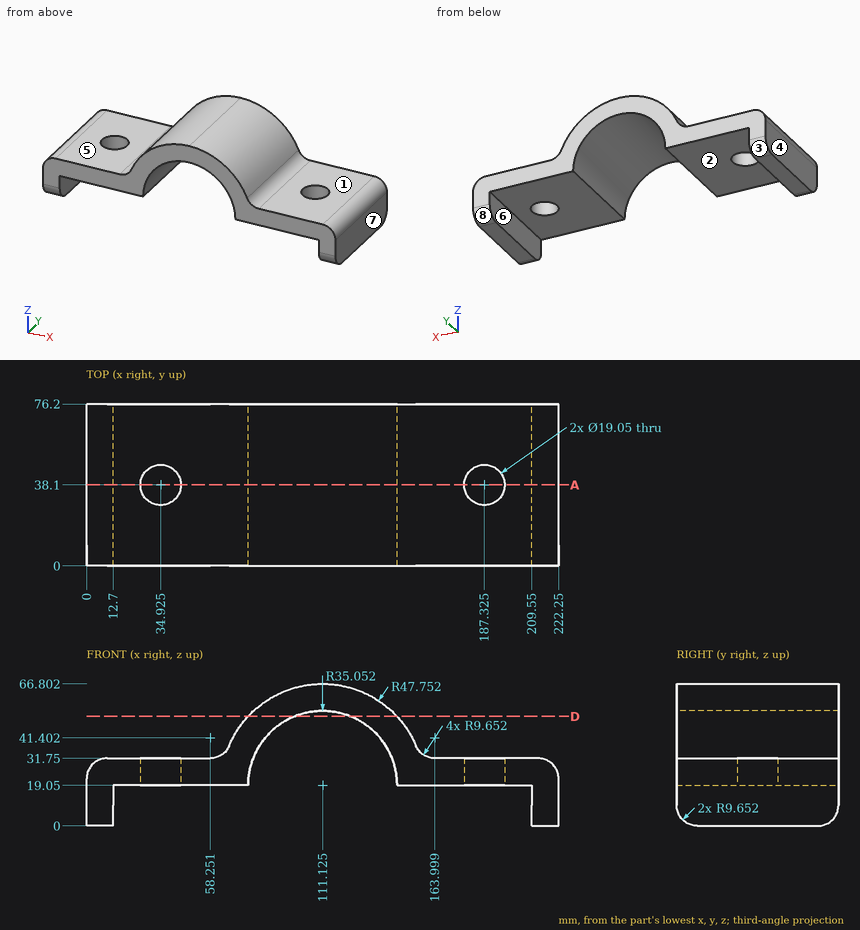
Job drawing, mm, ordinate dimensions from the low corner. One solid piece. A direction names the side the tool comes from. Coordinates: 2 decimals unless noted, no trailing zeros. Order: outer loops, then holes, each group sorted by start corner. A loop starts at its lowest first (then second) coordinate and runs counter-clockwise, first axis right, second up. Notation, with made-up numbers: (-19.75, 85) -> (25.25, 85) arc R34 cw to (25.25, 121) -> close; hole circle Ø3 at (64, 50.25). An arc over 180 degrees is marked (long way). Put each result on its own line as item: value. Start each with the question number.
(1) Pin check, flat tips, straight feed: pin 1 Ø3 at (y, z) = (17.5, 39) entering from +X; pin 2 Ø1 at (y, z) = (11, 30) entering from +X; pin 3 Ø2 at (x, y) = (115.5, 25.5) entering from -Z. Stop position of each tip, or through.
(2) Mould opens along X. For the marked faces 6, 7 and 8 say: pulls with the +X half, pulls with the -X half, needs draft (parallel to the pull), parting line crosses it, or undercut.
(3) Band-saw the part on A-A (y = 38.1). Count the separate pieces of the cut face and the enclosed holes in it, then the cut area to 3 significant figures.
(4) Which spindle directions (+Z, -Z, +X, -X, +Y, -Y) get a long thin tool onto all of the face, cutting with end or side? Do the marked faces 1, 2, 3, 4 and 5. Say none if no direction does.
(5) Probe line 1 along X through (y, z) = (39, 27.5) (1 decimal); line 2 along X through (y, z) = (38.1, 23.5); line 3 along Z through (x, y) = (28, 4.5). List the from-to ranges inside material, lowest first. Write a range as [from, to].
(6) Band-saw the part on D-D (z = 51.5). Give the cut face in (x, y), then the cut area to 3 significant figures.
Determined:
1. pin 1: stops at x = 155.17
1. pin 2: stops at x = 218.79
1. pin 3: stops at z = 53.69
2. face 6: undercut
2. face 7: pulls with the +X half
2. face 8: needs draft
3. separate pieces: 3
3. enclosed holes: 0
3. area: 3,250 mm²
4. face 1: +Z, +X, +Y, -Y
4. face 2: -Z, +Y, -Y
4. face 3: -Z, +X, -X, +Y
4. face 4: +Z, -Z, -X, +Y, -Y
4. face 5: +Z, -X, +Y, -Y
5. line 1: x = [1.7, 25.4], [44.4, 77.1], [145.1, 177.8], [196.8, 220.6]
5. line 2: x = [0.1, 25.4], [44.45, 76.36], [145.89, 177.8], [196.85, 222.15]
5. line 3: z = [19.05, 31.75]
6. outline: (76.09, 0) -> (97.87, 0) -> (97.87, 76.2) -> (76.09, 76.2) -> close; (124.38, 0) -> (146.16, 0) -> (146.16, 76.2) -> (124.38, 76.2) -> close
6. area: 3,320 mm²
